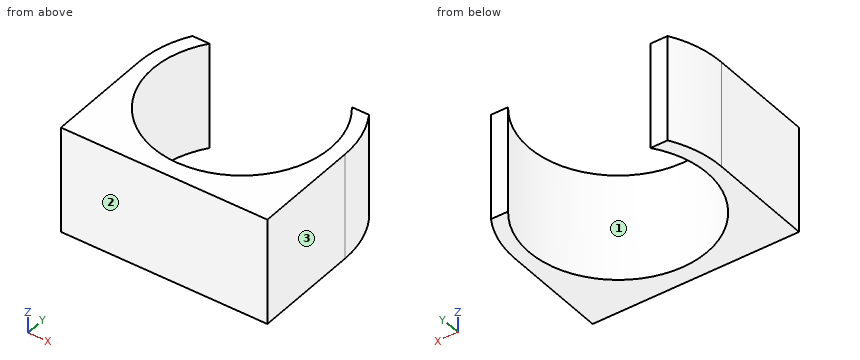
from build123d import *

# Parameters (mm, degrees)
F1_DEPTH = 15


with BuildPart() as f1:
    # F0 (on Top) → F1 (new body)
    with BuildSketch(Plane.XY):
        with BuildLine():
            ThreePointArc((24.5, 22.5), (14.5, 2.5), (4.5, 22.5))
            Line((4.5, 22.5), (2.090326, 22.5))
            ThreePointArc((2.090326, 22.5), (0.532354, 18.892925), (0, 15))
            Line((0, 15), (0, 0))
            Line((0, 0), (29, 0))
            Line((29, 0), (29, 15))
            ThreePointArc((29, 15), (28.467646, 18.892925), (26.909674, 22.5))
            Line((26.909674, 22.5), (24.5, 22.5))
        make_face()
    extrude(amount=F1_DEPTH)


solid = f1.part
Could you check a few things on this model? Use its own coordinates, in mm. Face numbers are marked on the shaded views. Round coordinates to 2 decimals unless told otherwise and drop trailing zeros. Write each loop counter-clockwise with the first axis right and the second up, starting at its lowest first coordinate (ties: lowest second). Pieces come first, ordered by that corner, then holes. Notation, with made-up numbers: (10.25, 60) -> (50.25, 60) arc R20 cw to (50.25, 79) -> close; hole circle Ø10 at (-3, 23). An arc over 180 degrees is marked (long way). Use a Markdown table: item, result.
1. We'd pull the mould along X, two halves only. Please class the marked faces 1, 2 and 3: +X half, -X half, draft (parallel to the pull), parting line (faces both ways), or undercut.
Answer key:
| item | result |
|---|---|
| face 1 | undercut |
| face 2 | draft |
| face 3 | +X half |
2. If we section it at B-B (z = 5.5): List the corners of the cut face in (x, y) for me.
Answer key:
| item | result |
|---|---|
| outline | (0, 0) -> (29, 0) -> (29, 15) arc R14.5 ccw to (26.91, 22.5) -> (24.5, 22.5) arc R12.5 cw (long way) to (4.5, 22.5) -> (2.09, 22.5) arc R14.5 ccw to (0, 15) -> close |
3. For pin 1 Ø5 at (x, z) = (16.5, 9) entering from -Y, with a flat end and sliding along its axis, tell me the tip position at first contact or that it passes through.
Answer key:
| item | result |
|---|---|
| pin 1 | stops at y = 0 |
4. Please list where these lines run through material, in increasing order: probe 1 along X at (y, z) = (15, 9.25); probe 2 along Y at (x, z) = (25.25, 2.25); probe 3 along X at (y, z) = (12.25, 7.25).
Answer key:
| item | result |
|---|---|
| probe 1 | x = 0 to 2, 27 to 29 |
| probe 2 | y = 0 to 8.62, 21.38 to 22.5 |
| probe 3 | x = 0 to 2.31, 26.69 to 29 |
5. If we section it at A-A (x = 2.5): List the corners of the cut face in (y, z) for me, then the cut area to 4 significant figures.
Answer key:
| item | result |
|---|---|
| outline | (0, 0) -> (11.5, 0) -> (11.5, 15) -> (0, 15) -> close; (18.5, 0) -> (22.5, 0) -> (22.5, 15) -> (18.5, 15) -> close |
| area | 232.5 mm^2 |
6. If we section it at D-D (x = 14.5): List the corners of the cut face in (y, z) for me.
Answer key:
| item | result |
|---|---|
| outline | (0, 0) -> (2.5, 0) -> (2.5, 15) -> (0, 15) -> close |
7. If we section it at C-C (y = 12.25): List the corners of the cut face in (x, z) for me, then the cut area to 3 significant figures.
Answer key:
| item | result |
|---|---|
| outline | (0, 0) -> (2.31, 0) -> (2.31, 15) -> (0, 15) -> close; (26.69, 0) -> (29, 0) -> (29, 15) -> (26.69, 15) -> close |
| area | 69.2 mm^2 |
